Here's how the part is built. I have some questions about the finished solid (model axes, mm). Round coordinates to 2 decimals unless told otherwise and drop trailing zeros. Write each loop counter-clockwise with the first axis right and the second up, starting at its lowest first coordinate (ties: lowest second). Pieces come first, ordered by that corner, then holes. Notation, with made-up numbers: (-22.75, -3.75) - (-12.75, -3.75) arc R23 ccw to (-12.75, 21.25) - close; hole circle Ø6 at (60.5, 67). An arc over 180 degrees is marked (long way). One line per item, written item: value. Start each with the question number.
Item 1: Imagine slicing it at A-A, the plane z = 5.5. Please give me the cut outline in (x, y).
Item 2: Imagine slicing it at C-C, the plane y = 37. Please give me the cut outline in (x, z), then the cut area to 3 significant figures.
Item 3: For P1, Ø0.5, axis at y = 14.5, z = 0.5, coming from the +X side; P2, Ø10, axis at x = -25, y = -6, coming from the +Z side, each with a flat end and sliding along its axis, tell me the tip position at first contact or that it passes through.
Item 4: If I drill on line 1 (Y direction, x = 33, z = 3.75); line 2 (Z direction, x = -4, y = -41.5), over which ranges is the centre line in solid material (lowest first)?
Item 5: Imagine slicing it at B-B, the plane x = 19.5. Please give me the cut outline in (y, z).
Item 6: Thinking about a two-plate mould opening in Y: for faces 1 (the face through (-19, 60.118, 3)), 2 (the face through (-19, -1, 0)), 3 (the face through (-27, -1, 1)), which applies, released by +Y, released by -Y, zero draft, split by the parting line, or undercut?
```python
from build123d import *

# Parameters (mm, degrees)
F0_W     = 140
F0_H     = 124
F1_DEPTH = 7
F2_T     = -1
F3_W     = 122
F3_H     = 6
F4_DEPTH = 1
F5_W     = 122
F5_H     = 6
F6_DEPTH = 1
F7_W     = 15
F7_H     = 122
F8_DEPTH = 1


with BuildPart() as f1:
    # F0 (on Top) → F1 (new body)
    with BuildSketch(Plane.XY):
        with Locations((-18.4690234582, -1.8815491349)):
            Rectangle(F0_W, F0_H)
    extrude(amount=F1_DEPTH)

    # F2
    f2_openings = [f1.faces().sort_by_distance(p)[0] for p in [
        (-18.469023, -1.881549, 7),
    ]]
    offset(amount=F2_T, openings=f2_openings)

    # F3 (on face) → F4 (cut)
    with BuildSketch(Plane(origin=(-88.4690234582, 0, 0), x_dir=(0, -1, 0), z_dir=(-1, 0, 0))):
        with Locations((1.8815491349, 4)):
            Rectangle(F3_W, F3_H)
    extrude(amount=-F4_DEPTH, mode=Mode.SUBTRACT)

    # F5 (on face) → F6 (cut)
    with BuildSketch(Plane.YZ.offset(51.5309765418)):
        with Locations((-1.8815491349, 4)):
            Rectangle(F5_W, F5_H)
    extrude(amount=-F6_DEPTH, mode=Mode.SUBTRACT)

    # F7 (on face) → F8 (cut)
    with BuildSketch(Plane.XY.offset(1)):
        with Locations((44.0309765418, -1.8815491349)):
            Rectangle(F7_W, F7_H)
    extrude(amount=-F8_DEPTH, mode=Mode.SUBTRACT)


solid = f1.part
```
Values follow:
1. outline: (-88.47, -63.88) - (51.53, -63.88) - (51.53, -62.88) - (-88.47, -62.88) - close; (-88.47, 59.12) - (51.53, 59.12) - (51.53, 60.12) - (-88.47, 60.12) - close
2. outline: (-88.47, 0) - (36.53, 0) - (36.53, 1) - (-88.47, 1) - close
2. area: 125 mm^2
3. P1: stops at x = 36.53
3. P2: stops at z = 1
4. line 1: y = -63.88 to -62.88, 59.12 to 60.12
4. line 2: z = 0 to 1
5. outline: (-63.88, 0) - (60.12, 0) - (60.12, 7) - (59.12, 7) - (59.12, 1) - (-62.88, 1) - (-62.88, 7) - (-63.88, 7) - close
6. face 1: released by +Y
6. face 2: zero draft
6. face 3: undercut
